Read the model definition and answer for the solid it produces. Units are mm, in the model's axes. Face numbers are marked on the shaded views. A direction names the side the tool comes from. Give positions to 0.01 mm unless a question says otherwise; leave off trailing zeros. Write each loop counter-clockwise with the first axis right and the second up, starting at its lowest first coordinate (ties: lowest second). Pieces come first, ordered by that corner, then holes. Notation, with made-up numbers: (14, -27) -> (32, -27) arc R28 cw to (32, 4) -> close; hole circle Ø7 at (-9, 1.25). An arc over 180 degrees is marked (long way). Use a Markdown table: item, result.
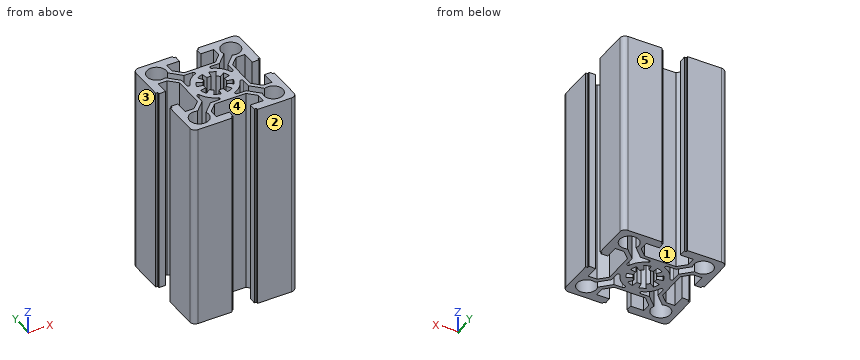
from build123d import *

# Parameters (mm, degrees)
EXTRUDE_1_DEPTH = 100


with BuildPart() as part:
    # 草图1 → 凸台-拉伸1 (new body)
    with BuildSketch(Plane.XY):
        with BuildLine():
            Line((-4.765977756, 26.059817672), (-21.165977756, 26.059817672))
            ThreePointArc((-21.165977756, 26.059817672), (-22.933744709, 25.327584625), (-23.665977756, 23.559817672))
            Line((-23.665977756, 23.559817672), (-23.665977756, 7.159817672))
            Line((-23.665977756, 7.159817672), (-22.965977756, 7.159817672))
            ThreePointArc((-22.965977756, 7.159817672), (-22.753845722, 7.071949706), (-22.665977756, 6.859817672))
            Line((-22.665977756, 6.859817672), (-22.665977756, 6.159817672))
            Line((-22.665977756, 6.159817672), (-19.465977756, 6.159817672))
            Line((-19.465977756, 6.159817672), (-19.465977756, 12.359817672))
            Line((-19.465977756, 12.359817672), (-15.198567937, 12.359817672))
            Line((-15.198567937, 12.359817672), (-11.398567937, 8.559817672))
            Line((-11.398567937, 8.559817672), (-11.398567937, 1.059817672))
            Line((-11.398567937, 1.059817672), (-11.398567937, -6.440182328))
            Line((-11.398567937, -6.440182328), (-15.198567937, -10.240182328))
            Line((-15.198567937, -10.240182328), (-19.465977756, -10.240182328))
            Line((-19.465977756, -10.240182328), (-19.465977756, -4.040182328))
            Line((-19.465977756, -4.040182328), (-22.665977756, -4.040182328))
            Line((-22.665977756, -4.040182328), (-22.665977756, -4.740182328))
            ThreePointArc((-22.665977756, -4.740182328), (-22.753845722, -4.952314363), (-22.965977756, -5.040182328))
            Line((-22.965977756, -5.040182328), (-23.665977756, -5.040182328))
            Line((-23.665977756, -5.040182328), (-23.665977756, -21.440182328))
            ThreePointArc((-23.665977756, -21.440182328), (-22.933744709, -23.207949281), (-21.165977756, -23.940182328))
            Line((-21.165977756, -23.940182328), (-4.765977756, -23.940182328))
            Line((-4.765977756, -23.940182328), (-4.765977756, -23.240182328))
            ThreePointArc((-4.765977756, -23.240182328), (-4.67810979, -23.028050294), (-4.465977756, -22.940182328))
            Line((-4.465977756, -22.940182328), (-3.765977756, -22.940182328))
            Line((-3.765977756, -22.940182328), (-3.765977756, -19.740182328))
            Line((-3.765977756, -19.740182328), (-9.965977756, -19.740182328))
            Line((-9.965977756, -19.740182328), (-9.965977756, -15.472772509))
            Line((-9.965977756, -15.472772509), (-6.165977756, -11.672772509))
            Line((-6.165977756, -11.672772509), (1.334022244, -11.672772509))
            Line((1.334022244, -11.672772509), (8.834022244, -11.672772509))
            Line((8.834022244, -11.672772509), (12.634022244, -15.472772509))
            Line((12.634022244, -15.472772509), (12.634022244, -19.740182328))
            Line((12.634022244, -19.740182328), (6.434022244, -19.740182328))
            Line((6.434022244, -19.740182328), (6.434022244, -22.940182328))
            Line((6.434022244, -22.940182328), (7.134022244, -22.940182328))
            ThreePointArc((7.134022244, -22.940182328), (7.346154278, -23.028050294), (7.434022244, -23.240182328))
            Line((7.434022244, -23.240182328), (7.434022244, -23.940182328))
            Line((7.434022244, -23.940182328), (23.834022244, -23.940182328))
            ThreePointArc((23.834022244, -23.940182328), (25.601789197, -23.207949281), (26.334022244, -21.440182328))
            Line((26.334022244, -21.440182328), (26.334022244, -5.040182328))
            Line((26.334022244, -5.040182328), (25.634022244, -5.040182328))
            ThreePointArc((25.634022244, -5.040182328), (25.42189021, -4.952314363), (25.334022244, -4.740182328))
            Line((25.334022244, -4.740182328), (25.334022244, -4.040182328))
            Line((25.334022244, -4.040182328), (22.134022244, -4.040182328))
            Line((22.134022244, -4.040182328), (22.134022244, -10.240182328))
            Line((22.134022244, -10.240182328), (17.866612425, -10.240182328))
            Line((17.866612425, -10.240182328), (14.066612425, -6.440182328))
            Line((14.066612425, -6.440182328), (14.066612425, 1.059817672))
            Line((14.066612425, 1.059817672), (14.066612425, 8.559817672))
            Line((14.066612425, 8.559817672), (17.866612425, 12.359817672))
            Line((17.866612425, 12.359817672), (22.134022244, 12.359817672))
            Line((22.134022244, 12.359817672), (22.134022244, 6.159817672))
            Line((22.134022244, 6.159817672), (25.334022244, 6.159817672))
            Line((25.334022244, 6.159817672), (25.334022244, 6.859817672))
            ThreePointArc((25.334022244, 6.859817672), (25.42189021, 7.071949706), (25.634022244, 7.159817672))
            Line((25.634022244, 7.159817672), (26.334022244, 7.159817672))
            Line((26.334022244, 7.159817672), (26.334022244, 23.559817672))
            ThreePointArc((26.334022244, 23.559817672), (25.601789197, 25.327584625), (23.834022244, 26.059817672))
            Line((23.834022244, 26.059817672), (7.434022244, 26.059817672))
            Line((7.434022244, 26.059817672), (7.434022244, 25.359817672))
            ThreePointArc((7.434022244, 25.359817672), (7.346154278, 25.147685637), (7.134022244, 25.059817672))
            Line((7.134022244, 25.059817672), (6.434022244, 25.059817672))
            Line((6.434022244, 25.059817672), (6.434022244, 21.859817672))
            Line((6.434022244, 21.859817672), (12.634022244, 21.859817672))
            Line((12.634022244, 21.859817672), (12.634022244, 17.592407853))
            Line((12.634022244, 17.592407853), (8.834022244, 13.792407853))
            Line((8.834022244, 13.792407853), (1.334022244, 13.792407853))
            Line((1.334022244, 13.792407853), (-6.165977756, 13.792407853))
            Line((-6.165977756, 13.792407853), (-9.965977756, 17.592407853))
            Line((-9.965977756, 17.592407853), (-9.965977756, 21.859817672))
            Line((-9.965977756, 21.859817672), (-3.765977756, 21.859817672))
            Line((-3.765977756, 21.859817672), (-3.765977756, 25.059817672))
            Line((-3.765977756, 25.059817672), (-4.465977756, 25.059817672))
            ThreePointArc((-4.465977756, 25.059817672), (-4.67810979, 25.147685637), (-4.765977756, 25.359817672))
            Line((-4.765977756, 25.359817672), (-4.765977756, 26.059817672))
        make_face()
        with BuildLine():
            Line((-9.765977756, 5.391903688), (-9.765977756, 9.61423326))
            Line((-9.765977756, 9.61423326), (-14.745444053, 14.593699556))
            ThreePointArc((-14.745444053, 14.593699556), (-19.718668949, 22.112508865), (-12.19985964, 17.139283969))
            Line((-12.19985964, 17.139283969), (-7.220393344, 12.159817672))
            Line((-7.220393344, 12.159817672), (-2.998063772, 12.159817672))
            ThreePointArc((-2.998063772, 12.159817672), (-2.29011, 11.688982743), (-2.450583757, 10.854038285))
            ThreePointArc((-2.450583757, 10.854038285), (-6.090598958, 8.484438874), (-8.460198369, 4.844423672))
            ThreePointArc((-8.460198369, 4.844423672), (-9.295142827, 4.683949916), (-9.765977756, 5.391903688))
        make_face(mode=Mode.SUBTRACT)
        with BuildLine():
            Line((-3.11053962, -5.591939227), (-1.499385944, -3.180677351))
            ThreePointArc((-1.499385944, -3.180677351), (-2.27222234, -2.546426912), (-2.906472779, -1.773590517))
            Line((-2.906472779, -1.773590517), (-5.317734654, -3.384744192))
            ThreePointArc((-5.317734654, -3.384744192), (-6.057014016, -2.001649787), (-6.512259999, -0.500904904))
            Line((-6.512259999, -0.500904904), (-3.667982686, 0.06485703))
            ThreePointArc((-3.667982686, 0.06485703), (-3.765977756, 1.059817672), (-3.667982686, 2.054778314))
            Line((-3.667982686, 2.054778314), (-6.512259999, 2.620540248))
            ThreePointArc((-6.512259999, 2.620540248), (-6.057014016, 4.121285131), (-5.317734654, 5.504379536))
            Line((-5.317734654, 5.504379536), (-2.906472779, 3.89322586))
            ThreePointArc((-2.906472779, 3.89322586), (-2.27222234, 4.666062256), (-1.499385944, 5.300312695))
            Line((-1.499385944, 5.300312695), (-3.11053962, 7.71157457))
            ThreePointArc((-3.11053962, 7.71157457), (-1.727445215, 8.450853932), (-0.226700332, 8.906099915))
            Line((-0.226700332, 8.906099915), (0.339061602, 6.061822602))
            ThreePointArc((0.339061602, 6.061822602), (1.334022244, 6.159817672), (2.328982886, 6.061822602))
            Line((2.328982886, 6.061822602), (2.89474482, 8.906099915))
            ThreePointArc((2.89474482, 8.906099915), (4.395489703, 8.450853932), (5.778584108, 7.71157457))
            Line((5.778584108, 7.71157457), (4.167430432, 5.300312695))
            ThreePointArc((4.167430432, 5.300312695), (4.940266828, 4.666062256), (5.574517267, 3.89322586))
            Line((5.574517267, 3.89322586), (7.985779142, 5.504379536))
            ThreePointArc((7.985779142, 5.504379536), (8.725058504, 4.121285131), (9.180304487, 2.620540248))
            Line((9.180304487, 2.620540248), (6.336027174, 2.054778314))
            ThreePointArc((6.336027174, 2.054778314), (6.434022244, 1.059817672), (6.336027174, 0.06485703))
            Line((6.336027174, 0.06485703), (9.180304487, -0.500904904))
            ThreePointArc((9.180304487, -0.500904904), (8.725058504, -2.001649787), (7.985779142, -3.384744192))
            Line((7.985779142, -3.384744192), (5.574517267, -1.773590517))
            ThreePointArc((5.574517267, -1.773590517), (4.940266828, -2.546426912), (4.167430432, -3.180677351))
            Line((4.167430432, -3.180677351), (5.778584108, -5.591939227))
            ThreePointArc((5.778584108, -5.591939227), (4.395489703, -6.331218588), (2.89474482, -6.786464571))
            Line((2.89474482, -6.786464571), (2.328982886, -3.942187258))
            ThreePointArc((2.328982886, -3.942187258), (1.334022244, -4.040182328), (0.339061602, -3.942187258))
            Line((0.339061602, -3.942187258), (-0.226700332, -6.786464571))
            ThreePointArc((-0.226700332, -6.786464571), (-1.727445215, -6.331218588), (-3.11053962, -5.591939227))
        make_face(mode=Mode.SUBTRACT)
        with BuildLine():
            Line((12.434022244, 5.391903688), (12.434022244, 9.61423326))
            Line((12.434022244, 9.61423326), (17.413488541, 14.593699556))
            ThreePointArc((17.413488541, 14.593699556), (22.386713437, 22.112508865), (14.867904128, 17.139283969))
            Line((14.867904128, 17.139283969), (9.888437832, 12.159817672))
            Line((9.888437832, 12.159817672), (5.66610826, 12.159817672))
            ThreePointArc((5.66610826, 12.159817672), (4.958154488, 11.688982743), (5.118628245, 10.854038285))
            ThreePointArc((5.118628245, 10.854038285), (8.758643446, 8.484438874), (11.128242857, 4.844423672))
            ThreePointArc((11.128242857, 4.844423672), (11.963187315, 4.683949916), (12.434022244, 5.391903688))
        make_face(mode=Mode.SUBTRACT)
        with BuildLine():
            Line((-9.765977756, -3.272268344), (-9.765977756, -7.494597916))
            Line((-9.765977756, -7.494597916), (-14.745444053, -12.474064213))
            ThreePointArc((-14.745444053, -12.474064213), (-19.718668949, -19.992873522), (-12.19985964, -15.019648625))
            Line((-12.19985964, -15.019648625), (-7.220393344, -10.040182328))
            Line((-7.220393344, -10.040182328), (-2.998063772, -10.040182328))
            ThreePointArc((-2.998063772, -10.040182328), (-2.29011, -9.569347399), (-2.450583757, -8.734402941))
            ThreePointArc((-2.450583757, -8.734402941), (-6.090598958, -6.364803531), (-8.460198369, -2.724788329))
            ThreePointArc((-8.460198369, -2.724788329), (-9.295142827, -2.564314572), (-9.765977756, -3.272268344))
        make_face(mode=Mode.SUBTRACT)
        with BuildLine():
            Line((12.434022244, -3.272268344), (12.434022244, -7.494597916))
            Line((12.434022244, -7.494597916), (17.413488541, -12.474064213))
            ThreePointArc((17.413488541, -12.474064213), (22.386713437, -19.992873522), (14.867904128, -15.019648625))
            Line((14.867904128, -15.019648625), (9.888437832, -10.040182328))
            Line((9.888437832, -10.040182328), (5.66610826, -10.040182328))
            ThreePointArc((5.66610826, -10.040182328), (4.958154488, -9.569347399), (5.118628245, -8.734402941))
            ThreePointArc((5.118628245, -8.734402941), (8.758643446, -6.364803531), (11.128242857, -2.724788329))
            ThreePointArc((11.128242857, -2.724788329), (11.963187315, -2.564314572), (12.434022244, -3.272268344))
        make_face(mode=Mode.SUBTRACT)
    extrude(amount=EXTRUDE_1_DEPTH)


solid = part.part
Item 1: A cutting plane is placed at B-B (x = 19.5). Give the vertices of the cut face in (y, z), then the cut area to 3 significant figures.
Return value:
| item | result |
|---|---|
| outline | (-23.94, 0) -> (-21.33, 0) -> (-21.33, 100) -> (-23.94, 100) -> close; (-12.15, 0) -> (-10.24, 0) -> (-10.24, 100) -> (-12.15, 100) -> close; (12.36, 0) -> (14.27, 0) -> (14.27, 100) -> (12.36, 100) -> close; (23.45, 0) -> (26.06, 0) -> (26.06, 100) -> (23.45, 100) -> close |
| area | 906 mm^2 |
Item 2: A cutting plane is placed at A-A (y = 19). Give the vertices of the cut face in (x, z).
Return value:
| item | result |
|---|---|
| outline | (-23.67, 0) -> (-21.06, 0) -> (-21.06, 100) -> (-23.67, 100) -> close; (-11.87, 0) -> (-9.97, 0) -> (-9.97, 100) -> (-11.87, 100) -> close; (12.63, 0) -> (14.54, 0) -> (14.54, 100) -> (12.63, 100) -> close; (23.73, 0) -> (26.33, 0) -> (26.33, 100) -> (23.73, 100) -> close |
Item 3: Each of these flat-tipped pins is pushed along its axis until it touches: P1, Ø4, axis at x = -2.5, z = 30.5, coming from the -Y side; P2, Ø1, axis at x = -0.5, z = 23, coming from the -Y side; P3, Ø0.8, axis at y = -23.5, z = 53.5, coming from the +X side. Where does it stop, or does it pass through?
Return value:
| item | result |
|---|---|
| P1 | y = -22.94 |
| P2 | y = -11.67 |
| P3 | x = 25.7 |
Item 4: A tool of negligible diameter and unlimited length cuts with its end or side. For the marked faces 4 and 5, from which of +Z, -Z, +X, -X, +Y, -Y can it reach the whole face along a straight path? Write none if from no direction.
Return value:
| item | result |
|---|---|
| face 4 | +Z, -Z |
| face 5 | +Z, -Z, +X, -X, +Y |
Item 5: For a pull along Y with two mould halves and no side action, classify the marked faces 1, 2 and 3 as +Y half, -Y half, draft (parallel to the pull), parting line (faces both ways), or undercut.
Return value:
| item | result |
|---|---|
| face 1 | undercut |
| face 2 | -Y half |
| face 3 | draft |
Item 6: A cutting plane is placed at C-C (z = 69). Count the separate pieces of the cut face and the enclosed holes in it, then the cut area to 3 significant figures.
Return value:
| item | result |
|---|---|
| separate pieces | 1 |
| enclosed holes | 5 |
| area | 1,030 mm^2 |
Item 7: Straight lines are drawn through the part: line 1 along Y through (x, z) = (-16, 89); line 2 along Y through (x, z) = (19, 89); line 3 along X through (y, z) = (-9.5, 6). For each, find the intervals that lie inside material, in ascending order. Write a range as [from, to].
Return value:
| item | result |
|---|---|
| line 1 | [-23.94, -21.32], [-12.16, -10.24], [12.36, 14.28], [23.44, 26.06] |
| line 2 | [-23.94, -21.34], [-12.14, -10.24], [12.36, 14.26], [23.46, 26.06] |
| line 3 | [-23.67, -19.47], [-14.46, -11.77], [-2.26, 4.93], [14.44, 17.13], [22.13, 26.33] |
